Verification items for the finished model (mm, model axes). A direction names the side the tool comes from. Give positions to 0.01 mm unless a question says otherwise; leave off trailing zeros. Write each loop counter-clockwise with the first axis right and the second up, starting at its lowest first coordinate (ties: lowest second). Pieces come first, ordered by that corner, then holes.
from build123d import *

# Parameters (mm, degrees)
SKETCH1_W           = 60
SKETCH1_H           = 33
BOSS_EXTRUDE1_DEPTH = 3
SKETCH2_R           = 1.3
CUT_EXTRUDE1_DEPTH  = 3
BOSS_EXTRUDE2_START = 4
SKETCH3_R           = 2
SKETCH3_R_2         = 1.3
BOSS_EXTRUDE2_DEPTH = 4
FILLET1_R           = 1
CUT_EXTRUDE2_DEPTH  = 2
FILLET2_R           = 11
SKETCH5_W           = 9
SKETCH5_H           = 4.5
CUT_EXTRUDE3_DEPTH  = 35.471002306
FILLET3_R           = 1


with BuildPart() as part:
    # Sketch1 → Boss-Extrude1 (new body)
    with BuildSketch(Plane(origin=(0, 0, 0), x_dir=(1, 0, 0), z_dir=(0, 1, 0))):
        Rectangle(SKETCH1_W, SKETCH1_H)
    extrude(amount=BOSS_EXTRUDE1_DEPTH)

    # Sketch2 → Cut-Extrude1 (cut)
    with BuildSketch(Plane(origin=(0, 3, 0), x_dir=(1, 0, 0), z_dir=(0, 1, 0))):
        with Locations(Location((-16.75, 9, 0), (0, 0, 270))):
            Circle(SKETCH2_R)
        with Locations(Location((16.75, 9, 0), (0, 0, 270))):
            Circle(SKETCH2_R)
        with Locations(Location((-16.75, -9, 0), (0, 0, 270))):
            Circle(SKETCH2_R)
        with Locations(Location((16.75, -9, 0), (0, 0, 270))):
            Circle(SKETCH2_R)
    extrude(amount=-CUT_EXTRUDE1_DEPTH, mode=Mode.SUBTRACT)

    # Sketch3 → Boss-Extrude2 (add)
    # profile 1 of 4: a face of its own
    with BuildSketch(Plane(origin=(0, 3, 0), x_dir=(1, 0, 0), z_dir=(0, 1, 0)).offset(BOSS_EXTRUDE2_START)):
        with Locations(Location((-16.75, 9, 0), (0, 0, 270))):
            Circle(SKETCH3_R)
        with Locations(Location((-16.75, 9, 0), (0, 0, 270))):
            Circle(SKETCH3_R_2, mode=Mode.SUBTRACT)
    # profile 2 of 4: a face of its own
    with BuildSketch(Plane(origin=(0, 3, 0), x_dir=(1, 0, 0), z_dir=(0, 1, 0)).offset(BOSS_EXTRUDE2_START)):
        with Locations(Location((-16.75, -9, 0), (0, 0, 270))):
            Circle(SKETCH3_R)
        with Locations(Location((-16.75, -9, 0), (0, 0, 270))):
            Circle(SKETCH3_R_2, mode=Mode.SUBTRACT)
    # profile 3 of 4: a face of its own
    with BuildSketch(Plane(origin=(0, 3, 0), x_dir=(1, 0, 0), z_dir=(0, 1, 0)).offset(BOSS_EXTRUDE2_START)):
        with Locations(Location((16.75, -9, 0), (0, 0, 270))):
            Circle(SKETCH3_R)
        with Locations(Location((16.75, -9, 0), (0, 0, 270))):
            Circle(SKETCH3_R_2, mode=Mode.SUBTRACT)
    # profile 4 of 4: a face of its own
    with BuildSketch(Plane(origin=(0, 3, 0), x_dir=(1, 0, 0), z_dir=(0, 1, 0)).offset(BOSS_EXTRUDE2_START)):
        with Locations(Location((16.75, 9, 0), (0, 0, 270))):
            Circle(SKETCH3_R)
        with Locations(Location((16.75, 9, 0), (0, 0, 270))):
            Circle(SKETCH3_R_2, mode=Mode.SUBTRACT)
    extrude(amount=-BOSS_EXTRUDE2_DEPTH)

    # Fillet1
    fillet1_edges = [part.edges().sort_by_distance(p)[0] for p in [
        (-16.75, 3, -11),
        (-16.75, 3, 7),
        (16.75, 3, 7),
        (16.75, 3, -11),
    ]]
    fillet(fillet1_edges, radius=FILLET1_R)

    # Sketch4 → Cut-Extrude2 (cut)
    with BuildSketch(Plane.XZ):
        Polygon((-15.508696921, 6.85), (-14.267393842, 9), (-15.508696921, 11.15), (-17.991303079, 11.15), (-19.232606158, 9), (-17.991303079, 6.85), align=None)
        Polygon((17.991303079, 6.85), (15.508696921, 6.85), (14.267393842, 9), (15.508696921, 11.15), (17.991303079, 11.15), (19.232606158, 9), align=None)
        Polygon((15.508696921, -6.85), (14.267393842, -9), (15.508696921, -11.15), (17.991303079, -11.15), (19.232606158, -9), (17.991303079, -6.85), align=None)
        Polygon((-17.991303079, -6.85), (-15.508696921, -6.85), (-14.267393842, -9), (-15.508696921, -11.15), (-17.991303079, -11.15), (-19.232606158, -9), align=None)
    extrude(amount=-CUT_EXTRUDE2_DEPTH, mode=Mode.SUBTRACT)

    # Fillet2
    fillet2_edges = [part.edges().sort_by_distance(p)[0] for p in [
        (-30, 1.5, -16.5),
        (30, 1.5, -16.5),
        (30, 1.5, 16.5),
        (-30, 1.5, 16.5),
    ]]
    fillet(fillet2_edges, radius=FILLET2_R)

    # Sketch5 → Cut-Extrude3 (cut, through all)
    with BuildSketch(Plane(origin=(0, 3, 0), x_dir=(1, 0, 0), z_dir=(0, 1, 0))):
        with Locations((-7.5, 4.25)):
            Rectangle(SKETCH5_W, SKETCH5_H)
        with Locations((7.5, 4.25)):
            Rectangle(SKETCH5_W, SKETCH5_H)
        with Locations((7.5, -4.25)):
            Rectangle(SKETCH5_W, SKETCH5_H)
        with Locations((-7.5, -4.25)):
            Rectangle(SKETCH5_W, SKETCH5_H)
    extrude(amount=-CUT_EXTRUDE3_DEPTH, mode=Mode.SUBTRACT)

    # Fillet3
    fillet3_edges = [part.edges().sort_by_distance(p)[0] for p in [
        (-12, 1.5, -2),
        (-12, 1.5, -6.5),
        (-3, 1.5, -6.5),
        (-3, 1.5, -2),
        (3, 1.5, -6.5),
        (12, 1.5, -6.5),
        (12, 1.5, -2),
        (3, 1.5, -2),
        (12, 1.5, 2),
        (12, 1.5, 6.5),
        (3, 1.5, 6.5),
        (3, 1.5, 2),
        (-3, 1.5, 6.5),
        (-12, 1.5, 6.5),
        (-12, 1.5, 2),
        (-3, 1.5, 2),
    ]]
    fillet(fillet3_edges, radius=FILLET3_R)


solid = part.part
Item 1: Scan lines: line 1 along X through (y, z) = (4.15, 9); line 2 along X through (y, z) = (2.5, -8); line 3 along Z through (x, y) = (14.5, 1.5). Record each from-to range of solid material in increasing order.
Answer key:
line 1: x = -18.75 to -18.05, -15.45 to -14.75, 14.75 to 15.45, 18.05 to 18.75
line 2: x = -29.71 to -17.58, -15.92 to 15.92, 17.58 to 29.71
line 3: z = -16.5 to -9.4, -8.6 to 8.6, 9.4 to 16.5
Item 2: Release check for a two-part mould opening along Y. For faces 5 (the face through (0, 3, 0)), 6 (the face through (-3, 2, -4)) record: released by +Y, released by -Y, zero draft, split by the parting line, or undercut.
Answer key:
face 5: released by +Y
face 6: zero draft
Item 3: Sectioned sample at B-B on x = -16.75. State how many separate pieces and enclosed holes the cut face has, then the cut area to 3 significant figures.
Answer key:
separate pieces: 3
enclosed holes: 0
area: 88.7 mm2
Item 4: Set-up check for faces 1 (the face through (-14.767, 5.521, 8.74)), 2 (the face through (-26.863, 1.521, -13.192)), 3 (the face through (18.62, 0.99, -7.94)), 4 (the face through (-8, 2, -2)): record each of +Z, -Z, +X, -X, +Y, -Y from which the full face is reachable in a straight line by a thin tool's end or side.
Answer key:
face 1: +Y
face 2: -Z, -X, +Y, -Y
face 3: -Y
face 4: +Y, -Y
Item 5: Sectioned sample at A-A on y = 4.75. Record the cut outline in (x, z).
Answer key:
outline: circle Ø4 at (-16.75, -9); circle Ø4 at (-16.75, 9); circle Ø4 at (16.75, -9); circle Ø4 at (16.75, 9); hole circle Ø2.6 at (-16.75, -9); hole circle Ø2.6 at (-16.75, 9); hole circle Ø2.6 at (16.75, -9); hole circle Ø2.6 at (16.75, 9)
Item 6: Depth check by flat-ended pin: pin 1 (1 mm diameter, centred on y = 1.5, z = 9.5, fed in from +X). Enter the tip coordinate at first touch or a pass-through.
Answer key:
pin 1: stops at x = 29.43
Item 7: Sectioned sample at D-D on x = 13. Record the cut outline in (y, z).
Answer key:
outline: (0, -16.5) - (3, -16.5) - (3, 16.5) - (0, 16.5) - close
